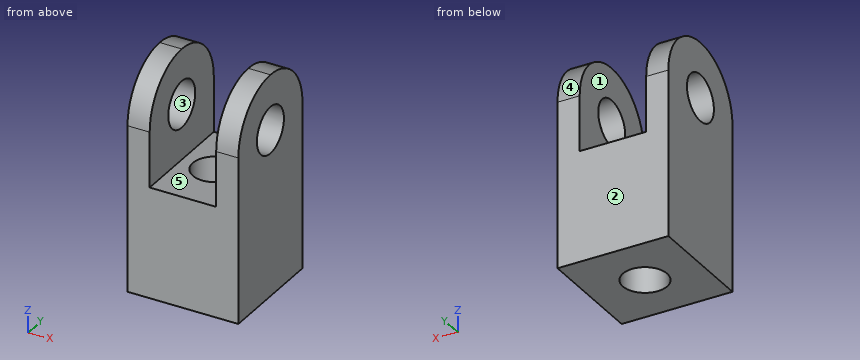
from build123d import *

# Parameters (mm, degrees)
SKETCH_1_W          = 10
SKETCH_1_H          = 10
SKETCH_1_R          = 2
EXTRUDE_1_DEPTH     = 10
SKETCH_2_W          = 2
SKETCH_2_H          = 10
EXTRUDE_2_DEPTH     = 10
SKETCH_3_R          = 2.1
CUT_EXTRUDE_1_DEPTH = 10
FILLET_1_R          = 5


with BuildPart() as part:
    # ｽｹｯﾁ1 → ﾎﾞｽ - 押し出し1 (new body)
    with BuildSketch(Plane.XY):
        Rectangle(SKETCH_1_W, SKETCH_1_H)
        Circle(SKETCH_1_R, mode=Mode.SUBTRACT)
    extrude(amount=EXTRUDE_1_DEPTH)

    # ｽｹｯﾁ2 → ﾎﾞｽ - 押し出し2 (add)
    with BuildSketch(Plane.XY.offset(10)):
        with Locations((-4, 0)):
            Rectangle(SKETCH_2_W, SKETCH_2_H)
        with Locations((4, 0)):
            Rectangle(SKETCH_2_W, SKETCH_2_H)
    extrude(amount=EXTRUDE_2_DEPTH)

    # ｽｹｯﾁ3 → ｶｯﾄ - 押し出し1 (cut)
    with BuildSketch(Plane(origin=(5, 0, 0), x_dir=(0, 0, -1), z_dir=(1, 0, 0))):
        with Locations(Location((-15, 0, 0), (0, 0, 90))):
            Circle(SKETCH_3_R)
    extrude(amount=-CUT_EXTRUDE_1_DEPTH, mode=Mode.SUBTRACT)

    # ﾌｨﾚｯﾄ1
    fillet_1_edges = [part.edges().sort_by_distance(p)[0] for p in [
        (4, -5, 20),
        (4, 5, 20),
        (-4, 5, 20),
        (-4, -5, 20),
    ]]
    fillet(fillet_1_edges, radius=FILLET_1_R - 0.0001)  # a hair under: the kernel refuses the full size


solid = part.part
Source: CAD feature listing. Evaluate the final solid. Frame: model axes, mm. Face numbers are marked on the shaded views. A direction names the side the tool comes from. Round coordinates to 2 decimals unless told otherwise and drop trailing zeros. Loops run counter-clockwise (first coordinate to the right, second up) from the corner with the lowest first, then second, coordinate; pieces in that order, holes last.
Q1. Section B-B, the plane z = 12.5. Return loops of the section in (x, y), plus the area to 3 significant figures.
Q2. First-contact query: P1, Ø1.8, axis at x = 1, y = -2, coming from the +Z side. Flat tip, straight axial feed; report the tip coordinate or a pass-through.
Q3. Ray query, line 1 (X direction, y = -2.75, z = 12); line 2 (Z direction, x = -3.8, y = 0); line 3 (Y direction, x = 0, z = 4). Return the intervals inside material, ascending.
Q4. Mould query, pull axis Y, two halves, no side actions, for the marked faces 3, 4 and 5. Classes: pulls with the +Y half, pulls with the -Y half, needs draft (parallel to the pull), parting line crosses it, or undercut.
Q5. Access query for the marked faces 1 and 2. Directions: +Z, -Z, +X, -X, +Y, -Y. A direction counts if a zero-diameter tool reaches every point of the face in a straight line with its end or side. Return the directions, or none.
Q6. Section A-A, the plane x = 0. Return loops of the section in (y, z), plus the area to 3 significant figures.
Q7. Section D-D, the plane z = 16.25. Return loops of the section in (x, y), plus the area to 3 significant figures.
Solutions:
1. outline: (-5, -5) - (-3, -5) - (-3, 5) - (-5, 5) - close; (3, -5) - (5, -5) - (5, 5) - (3, 5) - close
1. area: 40.0 mm2
2. P1: stops at z = 10
3. line 1: x = -5 to -3, 3 to 5
3. line 2: z = 0 to 12.9, 17.1 to 20
3. line 3: y = -5 to -2, 2 to 5
4. face 3: undercut
4. face 4: pulls with the +Y half
4. face 5: needs draft
5. face 1: +Z, +Y, -Y
5. face 2: +Z, -Z, +X, -X, +Y
6. outline: (-5, 0) - (-2, 0) - (-2, 10) - (-5, 10) - close; (2, 0) - (5, 0) - (5, 10) - (2, 10) - close
6. area: 60.0 mm2
7. outline: (-5, -4.84) - (-3, -4.84) - (-3, -1.69) - (-5, -1.69) - close; (-5, 1.69) - (-3, 1.69) - (-3, 4.84) - (-5, 4.84) - close; (3, -4.84) - (5, -4.84) - (5, -1.69) - (3, -1.69) - close; (3, 1.69) - (5, 1.69) - (5, 4.84) - (3, 4.84) - close
7. area: 25.2 mm2
